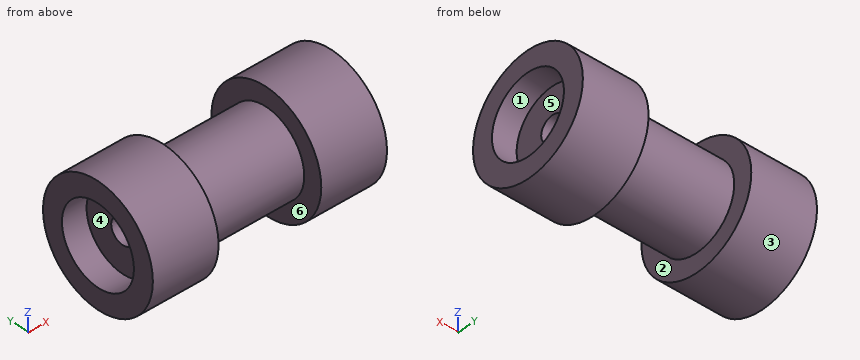
from build123d import *

# Parameters (mm, degrees)
SKETCH2_R          = 3
CUT_EXTRUDE1_DEPTH = 55.968172609


with BuildPart() as part:
    # Sketch1 → Revolve1 (revolve)
    with BuildSketch(Plane.XY, mode=Mode.PRIVATE) as revolve1_sk:
        Polygon((-12.5, 10), (12.5, 10), (12.5, 14.5), (28.5, 14.5), (28.5, 9.5), (22.5, 9.5), (22.5, 0), (-22.5, 0), (-22.5, 9.5), (-28.5, 9.5), (-28.5, 14.5), (-12.5, 14.5), align=None)
    revolve(revolve1_sk.sketch.rotate(Axis((-22.5, 0, 0), (1, 0, 0)), 180), axis=Axis((-22.5, 0, 0), (1, 0, 0)))

    # Sketch2 → Cut-Extrude1 (cut, through all)
    with BuildSketch(Plane.ZY.offset(22.5)):
        with Locations(Location((0, 0, 0), (0, 0, 270))):
            Circle(SKETCH2_R)
    extrude(amount=-CUT_EXTRUDE1_DEPTH, mode=Mode.SUBTRACT)


solid = part.part
Could you check a few things on this model? Use its own coordinates, in mm. Face numbers are marked on the shaded views. A direction names the side the tool comes from. Give positions to 0.01 mm unless a question says otherwise; leave off trailing zeros. Order: outer loops, then holes, each group sorted by start corner. A loop starts at its lowest first (then second) coordinate and runs counter-clockwise, first axis right, second up.
1. I need wall thicknesses on L1, parallel to X at y = 0.75, z = -10.75; L2, parallel to Z at x = -24.3, y = 0; L3, parallel to Z at x = 13, y = 0. Which ranges of each line are inside material? Lowest first, please.
2. We'd pull the mould along Z, two halves only. Please class the marked faces 1, 2 and 3: pulls with the +Z half, pulls with the -Z half, needs draft (parallel to the pull), parting line crosses it, or undercut.
3. Will these pins go through, and if not, where does the flat tip stop? P1, Ø6, axis at x = -1, y = 3.5, coming from the -Z side; P2, Ø1.5, axis at y = -7.5, z = 4, coming from the -X side; P3, Ø5, axis at x = -14.5, y = 3, coming from the -Z side.
4. For the marked faces 4, 5 and 6, which set-ups out of +Z, -Z, +X, -X, +Y, -Y let a thin tool reach every point of the face, with its end or its side?
5. Suppose I cut it at A-A (z = 0). List the corners of the cut face in (x, y) for me, plus the area to 3 significant figures.
6. Suppose I cut it at D-D (y = -7). List the corners of the cut face in (x, z) for me.
7. Suppose I cut it at C-C (x = 5.5). List the corners of the cut face in (y, z) for me, plus the area to 3 significant figures.
Solved:
1. L1: x = -28.5 to -12.5, 12.5 to 28.5
1. L2: z = -14.5 to -9.5, 9.5 to 14.5
1. L3: z = -14.5 to -3, 3 to 14.5
2. face 1: undercut
2. face 2: needs draft
2. face 3: parting line crosses it
3. P1: stops at z = -9.99
3. P2: stops at x = -22.5
3. P3: stops at z = -14.49
4. face 4: -X
4. face 5: +X
4. face 6: none
5. outline: (-28.5, -14.5) - (-12.5, -14.5) - (-12.5, -10) - (12.5, -10) - (12.5, -14.5) - (28.5, -14.5) - (28.5, -9.5) - (22.5, -9.5) - (22.5, -3) - (-22.5, -3) - (-22.5, -9.5) - (-28.5, -9.5) - close; (-28.5, 9.5) - (-22.5, 9.5) - (-22.5, 3) - (22.5, 3) - (22.5, 9.5) - (28.5, 9.5) - (28.5, 14.5) - (12.5, 14.5) - (12.5, 10) - (-12.5, 10) - (-12.5, 14.5) - (-28.5, 14.5) - close
5. area: 930 mm2
6. outline: (-28.5, -12.7) - (-12.5, -12.7) - (-12.5, -7.14) - (12.5, -7.14) - (12.5, -12.7) - (28.5, -12.7) - (28.5, -6.42) - (22.5, -6.42) - (22.5, 6.42) - (28.5, 6.42) - (28.5, 12.7) - (12.5, 12.7) - (12.5, 7.14) - (-12.5, 7.14) - (-12.5, 12.7) - (-28.5, 12.7) - (-28.5, 6.42) - (-22.5, 6.42) - (-22.5, -6.42) - (-28.5, -6.42) - close
7. outline: circle Ø20 at (0, 0); hole circle Ø6 at (0, 0)
7. area: 286 mm2
